from build123d import *

# Parameters (mm, degrees)
F0_W     = 1.4
F0_H     = 2
F1_DEPTH = 1.5
F0_H_2   = 1.1
F0_H_3   = 1.5
F2_DEPTH = 4
F3_DEPTH = 1.8
F4_W     = 1
F4_H     = 3.7
F5_DEPTH = 0.5
F6_R     = 0.5


with BuildPart() as f1:
    # F0 (on Top) → F1 (new body)
    with BuildSketch(Plane.XY):
        Polygon((2, -1.85), (0.7, -1.85), (0.7, -3.85), (5, -3.85), (5, 1.85), (2, 1.85), align=None)
        with Locations((0, -2.85)):
            Rectangle(F0_W, F0_H)
        Polygon((-0.7, -3.85), (-0.7, -1.85), (-2, -1.85), (-2, 1.85), (-5, 1.85), (-5, -3.85), align=None)
    extrude(amount=-F1_DEPTH)

    # F0 (on Top) → F2 (join)
    with BuildSketch(Plane.XY):
        with Locations((0, -1.3)):
            Rectangle(F0_W, F0_H_2)
        Rectangle(F0_W, F0_H_3)
        Polygon((-0.7, -1.85), (-0.7, -0.75), (-0.7, 0.75), (-0.7, 1.85), (-2, 1.85), (-2, -1.85), align=None)
        with Locations((0, 1.3)):
            Rectangle(F0_W, F0_H_2)
        Polygon((0.7, 0.75), (0.7, -0.75), (0.7, -1.85), (2, -1.85), (2, 1.85), (0.7, 1.85), align=None)
    extrude(amount=-F2_DEPTH)

    # F0 (on Top) → F3 (cut)
    with BuildSketch(Plane.XY):
        Rectangle(F0_W, F0_H_3)
        with Locations((0, 1.3)):
            Rectangle(F0_W, F0_H_2)
        with Locations((0, -1.3)):
            Rectangle(F0_W, F0_H_2)
        with Locations((0, -2.85)):
            Rectangle(F0_W, F0_H)
    extrude(amount=-F3_DEPTH, mode=Mode.SUBTRACT)

    # F4 (on face) → F5 (cut)
    with BuildSketch(Plane(origin=(0, 0, -4), x_dir=(1, 0, 0), z_dir=(0, 0, -1))):
        Rectangle(F4_W, F4_H)
    extrude(amount=-F5_DEPTH, mode=Mode.SUBTRACT)

    # F6
    f6_edges = [f1.edges().sort_by_distance(p)[0] for p in [
        (-2, 0, -4),
        (2, 0, -4),
    ]]
    fillet(f6_edges, radius=F6_R)


solid = f1.part
Geometry check sheet. Reference: the model listing, model coordinates, mm. A direction names the side the tool comes from. Round coordinates to 2 decimals unless told otherwise and drop trailing zeros. Loops run counter-clockwise (first coordinate to the right, second up) from the corner with the lowest first, then second, coordinate; pieces in that order, holes last.
Item 1: Cross-section at B-B on z = -0.8. Record the boundary of the cut face in (x, y), then the cut area to 3 significant figures.
Item 2: Mould release check, pull along X, two halves, no side actions. Record for faces 6 (the flat face through (2, 0, -2)), 7 (the flat face through (-3, -1, -1.5)), 8 (the flat face through (0, 0, -3.5)): pulls with the +X half, pulls with the -X half, needs draft (parallel to the pull), parting line crosses it, or undercut.
Item 3: Access from +Z, -Z, +X, -X, +Y, -Y to the whole of each face (thin tool, end or side, straight path). Record for faces 1 (the flat face through (0, -1.85, -3)), 2 (the flat face through (0.7, -1, -1)), 3 (the flat face through (5, -1, -1)), 4 (the flat face through (-3, -1, 0)), 5 (the flat face through (-2, 0, -2)).
Item 4: Gauge pin test, flat ends, axial feed: pin 1 (1.1 mm diameter, centred on x = 0, y = 0, fed in from -Z); pin 2 (1 mm diameter, centred on x = 3, z = -2.5, fed in from +Y); pin 3 (1 mm diameter, centred on y = 0, z = -2.5, fed in from +X); pin 4 (2 mm diameter, centred on y = 0, z = -3, fed in from -X). Record the tip position at first contact, or that the pin passes through.
Item 5: Thickness scan on line 1 (X direction, y = -0.95, z = -0.75); line 2 (X direction, y = 0.1, z = -1.55); line 3 (Z direction, x = -4, y = -3.4). Record the ranges inside material, lowest first.
Item 6: Cross-section at A-A on y = -2.65. Record the boundary of the cut face in (x, z), then the cut area to 3 significant figures.
Item 7: Cross-section at C-C on y = 0.2. Record the boundary of the cut face in (x, z).
Item 8: Cross-section at D-D on x = -3.5. Record the boundary of the cut face in (y, z), then the cut area to 3 significant figures.
Answer sheet:
1. outline: (-5, -3.85) - (-0.7, -3.85) - (-0.7, 1.85) - (-5, 1.85) - close; (0.7, -3.85) - (5, -3.85) - (5, 1.85) - (0.7, 1.85) - close
1. area: 49.0 mm2
2. face 6: pulls with the +X half
2. face 7: needs draft
2. face 8: undercut
3. face 1: -Z, +X, -X, -Y
3. face 2: +Z, +Y, -Y
3. face 3: +Z, -Z, +X, +Y, -Y
3. face 4: +Z, +X, -X, +Y, -Y
3. face 5: -Z, -X, +Y, -Y
4. pin 1: stops at z = -4
4. pin 2: passes through
4. pin 3: stops at x = 2
4. pin 4: stops at x = -2
5. line 1: x = -5 to -0.7, 0.7 to 5
5. line 2: x = -2 to -0.7, 0.7 to 2
5. line 3: z = -1.5 to 0
6. outline: (-5, -1.5) - (-0.7, -1.5) - (-0.7, 0) - (-5, 0) - close; (0.7, -1.5) - (5, -1.5) - (5, 0) - (0.7, 0) - close
6. area: 12.9 mm2
7. outline: (-5, -1.5) - (-2, -1.5) - (-2, -3.5) arc R0.5 ccw to (-1.5, -4) - (-0.5, -4) - (-0.5, -3.5) - (0.5, -3.5) - (0.5, -4) - (1.5, -4) arc R0.5 ccw to (2, -3.5) - (2, -1.5) - (5, -1.5) - (5, 0) - (0.7, 0) - (0.7, -1.8) - (-0.7, -1.8) - (-0.7, 0) - (-5, 0) - close
8. outline: (-3.85, -1.5) - (1.85, -1.5) - (1.85, 0) - (-3.85, 0) - close
8. area: 8.55 mm2
